Model file for the job. Use its own axes, mm. A direction names the side the tool comes from. Coordinates: 2 decimals unless noted, no trailing zeros. Order: outer loops, then holes, each group sorted by start corner. A loop starts at its lowest first (then second) coordinate and runs counter-clockwise, first axis right, second up. Notation, with made-up numbers: M 34,-12 L 48,-12 A27 cw 48,24 Z; hole C 56.5,-2.75 d1. An arc over 180 degrees is marked long. Return JSON: item names as keys, results as strings.
```python
from build123d import *

# Parameters (mm, degrees)
F0_W     = 7.2
F0_H     = 11
F0_R     = 3.3
F1_DEPTH = 23.4
F2_W     = 1.2
F2_H     = 4.8
F3_DEPTH = 11.001
F4_W     = 9.2
F4_H     = 9
F5_DEPTH = 11
F6_W     = 8.6
F6_H     = 4.5
F7_DEPTH = 6.5
F8_R     = 3.3
F9_DEPTH = 23.401


with BuildPart() as f1:
    # F0 (on Front) → F1 (new body)
    with BuildSketch(Plane.XZ):
        Rectangle(F0_W, F0_H)
        with Locations((0, -1.7)):
            Circle(F0_R, mode=Mode.SUBTRACT)
    extrude(amount=F1_DEPTH)

    # F2 (on face) → F3 (cut, through all)
    with BuildSketch(Plane.XY.offset(5.5)):
        with Locations((3, -2.4)):
            Rectangle(F2_W, F2_H)
        with Locations((-3, -2.4)):
            Rectangle(F2_W, F2_H)
    extrude(amount=-F3_DEPTH, mode=Mode.SUBTRACT)

    # F4 (on face) → F5 (join, through all)
    with BuildSketch(Plane.XY.offset(5.5)):
        with Locations((0, -9.3)):
            Rectangle(F4_W, F4_H)
    extrude(amount=-F5_DEPTH)

    # F6 (on face) → F7 (join)
    with BuildSketch(Plane.XY.offset(5.5)):
        with Locations((0, -21.15)):
            Rectangle(F6_W, F6_H)
    extrude(amount=-F7_DEPTH)

    # F8 (on face) → F9 (cut, through all)
    with BuildSketch(Plane.XZ.offset(23.4)):
        with Locations((0, -1.7)):
            Circle(F8_R)
    extrude(amount=-F9_DEPTH, mode=Mode.SUBTRACT)


solid = f1.part
```
Item 1: Drop flat-ended pins along their axis: pin 1 Ø1.1 at (x, z) = (3.5, -2.5) entering from +Y; pin 2 Ø3 at (y, z) = (-16.5, 0) entering from +X; pin 3 Ø2.5 at (y, z) = (-3, 2) entering from -X; pin 4 Ø1 at (x, z) = (1, -1.5) entering from +Y. Give the stop position or say it passes through.
Check result:
{"pin 1": "stops at y = -4.8", "pin 2": "stops at x = 3.6", "pin 3": "stops at x = -2.4", "pin 4": "passes through"}
Item 2: 3-axis set-ups, long thin cutter, end or side, ignore diameter. For faces 5 (the flat face through (-4.3, -21, 2)), 6 (the flat face through (4.3, -21, 2)), 7 (the flat face through (4, -13.8, 0)): which of +Z, -Z, +X, -X, +Y, -Y reach the whole face in a straight line?
Check result:
{"face 5": "+Z, -Z, -X, -Y", "face 6": "+Z, -Z, +X, -Y", "face 7": "+Z, -Z, +X"}
Item 3: Saw through at B-B (x = 0). Write the cut outline in (y, z).
Check result:
{"outline": "M -23.4,-5.5 L 0,-5.5 L 0,-5 L -23.4,-5 Z; M -23.4,1.6 L 0,1.6 L 0,5.5 L -23.4,5.5 Z"}
Item 4: Saw through at C-C (y = -18.25). Write the cut outline in (x, z), and give its area (3 significant figures).
Check result:
{"outline": "M -3.6,-5.5 L 3.6,-5.5 L 3.6,5.5 L -3.6,5.5 Z; hole C 0,-1.7 d6.6", "area": "45.0 mm2"}
Item 5: Saw through at A-A (z = -1.7). Write the cut outline in (x, y).
Check result:
{"outline": "M -4.6,-13.8 L -3.6,-13.8 L -3.6,-23.4 L -3.3,-23.4 L -3.3,-4.8 L -4.6,-4.8 Z; M 3.3,-23.4 L 3.6,-23.4 L 3.6,-13.8 L 4.6,-13.8 L 4.6,-4.8 L 3.3,-4.8 Z"}
Item 6: Pull direction Y, two halves, no side cores. Call faces 1 (the flat face through (-4, -13.8, 0)), 2 (the flat face through (0, -12, 5.5)), 3 (the flat face through (-4, -4.8, 0)), 4 (the flat face through (3.6, -17, -1)): +Y half, -Y half, draft (parallel to the pull), parting line (faces both ways), or undercut.
Check result:
{"face 1": "undercut", "face 2": "draft", "face 3": "+Y half", "face 4": "undercut"}
Item 7: Saw through at D-D (z = 3.25). Write the cut outline in (x, y), and give its area (3 significant figures).
Check result:
{"outline": "M -4.6,-13.8 L -3.6,-13.8 L -3.6,-18.9 L -4.3,-18.9 L -4.3,-23.4 L 4.3,-23.4 L 4.3,-18.9 L 3.6,-18.9 L 3.6,-13.8 L 4.6,-13.8 L 4.6,-4.8 L 2.4,-4.8 L 2.4,0 L -2.4,0 L -2.4,-4.8 L -4.6,-4.8 Z", "area": "181 mm2"}
Item 8: Wall check: line 1 (Y direction, x = -4, z = 1.75); line 2 (X direction, y = -8.25, z = -1.7); line 3 (Z direction, x = 0, y = -8). Give the ranges that are in metal, low to high.
Check result:
{"line 1": "y = -23.4 to -18.9, -13.8 to -4.8", "line 2": "x = -4.6 to -3.3, 3.3 to 4.6", "line 3": "z = -5.5 to -5, 1.6 to 5.5"}
